from build123d import *

# Parameters (mm, degrees)
F0_R     = 38.1
F1_DEPTH = 3.81
F2_R     = 38.1
F2_R_2   = 35.56
F3_DEPTH = 12.7
F4_R     = 5.08
F5_R     = 1.27
F6_DEPTH = 25.4
F7_R     = 3.175
F8_DEPTH = 1.27


with BuildPart() as f1:
    # F0 (on Top) → F1 (new body)
    with BuildSketch(Plane.XY):
        Circle(F0_R)
    extrude(amount=F1_DEPTH)

    # F2 (on face) → F3 (join)
    with BuildSketch(Plane.XY.offset(3.81)):
        Circle(F2_R)
        Circle(F2_R_2, mode=Mode.SUBTRACT)
    extrude(amount=F3_DEPTH)

    # F4
    f4_edges = [f1.edges().sort_by_distance(p)[0] for p in [
        (-35.56, 0, 3.81),
    ]]
    fillet(f4_edges, radius=F4_R)

    # F5 (on face) → F6 (cut)
    with BuildSketch(Plane.XY.offset(3.81)):
        Circle(F5_R)
    extrude(amount=-F6_DEPTH, mode=Mode.SUBTRACT)

    # F7 (on face) → F8 (cut)
    with BuildSketch(Plane(origin=(0, 0, 0), x_dir=(1, 0, 0), z_dir=(0, 0, -1))):
        Circle(F7_R)
    extrude(amount=-F8_DEPTH, mode=Mode.SUBTRACT)


solid = f1.part
Here's how the part is built. I have some questions about the finished solid (model axes, mm). A direction names the side the tool comes from. Give positions to 0.01 mm unless a question says otherwise; leave off trailing zeros. Order: outer loops, then holes, each group sorted by start corner. A loop starts at its lowest first (then second) coordinate and runs counter-clockwise, first axis right, second up. Notation, with made-up numbers: M 56.5,67.25 L 77.5,67.25 A16 cw 77.5,94.25 Z; hole C 61,-9.75 d6. An arc over 180 degrees is marked long. Answer as a JSON object with one key per item and string values. Group by question number.
1) We'd pull the mould along Y, two halves only. Please class faces 1 (the cylindrical face through (-0.17, 1.26, 2.56)), 2 (the flat face through (34, 11, 16.51)), 3 (the cylindrical face through (-30.235, -23.183, 8.139)): pulls with the +Y half, pulls with the -Y half, needs draft (parallel to the pull), parting line crosses it, or undercut.
2) On a 3-axis mill with a long thin cutter (end or side, diameter ignored), from which of +Z, -Z, +X, -X, +Y, -Y can I reach the whole of each face in a straight line? I mean faces 4 (the flat face through (1.4, 0.7, 1.27)), 5 (the flat face through (8, 1, 0)), 6 (the flat face through (0, -6, 3.81)). Say none if no direction works.
3) Suppose I cut it at C-C, the plane z = 15. Write out the boundary of the cut face in (x, y), plus the area to 3 significant figures.
4) Please list where these lines run through material, in increasing order: L1, parallel to Y at x = 0, z = 2.7; L2, parallel to Y at x = 0, z = 10.75; L3, parallel to X at y = 23, z = 12.5. Write a range as [from, to].
5) Suppose I cut it at A-A, the plane x = 0. Write out the boundary of the cut face in (y, z) (3 decimals).
6) I'm going to push flat-ended pins straight in: pin 1 Ø8 at (x, z) = (-11, 4.5) entering from +Y; pin 2 Ø8 at (x, y) = (20, 4) entering from +Z; pin 3 Ø3 at (x, y) = (0, 0.5) entering from -Z. Where does each tip first touch, or does it pass through?
Results found:
{
 "1": {"face 1": "undercut", "face 2": "needs draft", "face 3": "parting line crosses it"},
 "2": {"face 4": "-Z", "face 5": "-Z, +X, -X, +Y, -Y", "face 6": "+Z"},
 "3": {"outline": "C 0,0 d76.2; hole C 0,0 d71.12", "area": "588 mm²"},
 "4": {"L1": "[-38.1, -1.27], [1.27, 38.1]", "L2": "[-38.1, -35.56], [35.56, 38.1]", "L3": "[-30.37, -27.12], [27.12, 30.37]"},
 "5": {"outline": "M -38.1,0 L -3.175,0 L -3.175,1.27 L -1.27,1.27 L -1.27,3.81 L -30.48,3.81 A5.08 cw -35.56,8.89 L -35.56,16.51 L -38.1,16.51 Z; M 1.27,1.27 L 3.175,1.27 L 3.175,0 L 38.1,0 L 38.1,16.51 L 35.56,16.51 L 35.56,8.89 A5.08 cw 30.48,3.81 L 1.27,3.81 Z"},
 "6": {"pin 1": "y = 37.45", "pin 2": "z = 3.81", "pin 3": "z = 1.27"}
}
